Model file for the job. Use its own axes, mm. Face numbers are marked on the shaded views. A direction names the side the tool comes from. Round coordinates to 2 decimals unless told otherwise and drop trailing zeros. Loops run counter-clockwise (first coordinate to the right, second up) from the corner with the lowest first, then second, coordinate; pieces in that order, holes last. Notation, with made-up numbers: M 20,-2 L 44,-2 A27 cw 44,34 Z; hole C -18,85.5 d4. An arc over 180 degrees is marked long. Use a Markdown table: item, result. Add a question column.
Q1. Tool access for the marked faces 1 and 2: list every direction of +Z, -Z, +X, -X, +Y, -Y with a clear straight run to the whole face (end or side of a thin tool).
Q2. Mould opens along Y. For the marked faces 3, 4 and 5 say: +Y half, -Y half, draft (parallel to the pull), parting line (faces both ways), or undercut.
Q3. Probe line 1 (X direction, y = 1.3, z = 0); line 2 (Y direction, x = 1.5, z = -0.25); line 3 (Y direction, x = -1.7, z = 2.5). List the from-to ranges inside material, lowest first. Write a range as from..to.
Q4. Cut at B-B (z = 0). Give the cut face in (x, y) (3 decimals), plus the area to 3 significant figures.
Q5. Cut at C-C (y = 0.5). Give the cut face in (x, z).
Q6. Cut at D-D (z = -3). Give the cut face in (x, y).
Q7. Pin check, flat tips, straight feed: pin 1 (0.9 mm diameter, centred on x = 2, z = -3, fed in from +Y); pin 2 (2 mm diameter, centred on x = 1, y = 0.5, fed in from +Z). Stop position of each tip, or through.
Autodesk Inventor part; units mm, degrees
ref_plane "to_actuator_XY" through (0, 0, 0) normal (0, -1, 0) x (1, 0, 0)
ref_plane "to_actuator_YZ" through (0, 0, 0) normal (1, 0, 0) x (0, 0, 1)
ref_plane "to_actuator_ZX" through (0, 0, 0) normal (0, 0, 1) x (0, -1, 0)
sketch "Sketch_1" plane through (0, 0, 0) normal (0, 1, 0) x (-1, 0, 0)
  line L0 (2.2479, 3.5052) -> (-2.2479, 3.5052)
  line L1 (-2.2479, 3.5052) -> (-2.2479, -3.5052)
  line L2 (-2.2479, -3.5052) -> (2.2479, -3.5052)
  line L3 (2.2479, -3.5052) -> (2.2479, 3.5052)
extrude "Extrusion1" add sketch "Sketch_1" against normal blind 5.4102
sketch "Sketch_2" plane through (0, 0, 0) normal (0, 0, 1) x (1, 0, 0)
  line L0 (-2.2479, -0.7874) -> (-1.9456, 0)
  line L1 (-1.9456, 0) -> (1.9456, 0)
  line L2 (1.9456, 0) -> (2.2479, -0.7874)
  line L3 (2.2479, -0.7874) -> (2.2479, 0.127)
  line L4 (2.2479, 0.127) -> (-2.2479, 0.127)
  line L5 (-2.2479, 0.127) -> (-2.2479, -0.7874)
extrude "Extrusion2" cut sketch "Sketch_2" along normal mid plane 7.0104
sketch "Sketch_3" plane through (0, 0, 0) normal (1, 0, 0) x (0, 1, 0)
  line L0 (-0.7874, 3.5052) -> (0, 3.2029)
  line L1 (0, 3.2029) -> (0, -3.2029)
  line L2 (0, -3.2029) -> (-0.7874, -3.5052)
  line L3 (-0.7874, -3.5052) -> (0.127, -3.5052)
  line L4 (0.127, -3.5052) -> (0.127, 3.5052)
  line L5 (0.127, 3.5052) -> (-0.7874, 3.5052)
extrude "Extrusion3" cut sketch "Sketch_3" along normal mid plane 4.4958
sketch "Sketch_4" plane through (0, -0.9906, 0) normal (0, 1, 0) x (1, 0, 0)
  line L0 (-2.5256, 3.7556) -> (-2.5256, -3.7297)
  line L1 (-2.5256, -3.7297) -> (2.532, -3.7297)
  line L2 (2.532, -3.7297) -> (2.532, 3.7556)
  line L3 (2.532, 3.7556) -> (-2.5256, 3.7556)
  line L4 (-2.2479, 2.3368) -> (-2.2479, -2.3368)
  line L5 (-2.2479, -2.3368) -> (-1.0668, -2.3368)
  line L6 (-1.0668, -2.3368) -> (-1.0668, -3.5052)
  line L7 (-1.0668, -3.5052) -> (1.0668, -3.5052)
  line L8 (1.0668, -3.5052) -> (1.0668, -2.3368)
  line L9 (1.0668, -2.3368) -> (2.2479, -2.3368)
  line L10 (2.2479, -2.3368) -> (2.2479, 2.3368)
  line L11 (2.2479, 2.3368) -> (1.0668, 2.3368)
  line L12 (1.0668, 2.3368) -> (1.0668, 3.5052)
  line L13 (1.0668, 3.5052) -> (-1.0668, 3.5052)
  line L14 (-1.0668, 3.5052) -> (-1.0668, 2.3368)
  line L15 (-1.0668, 2.3368) -> (-2.2479, 2.3368)
extrude "Extrusion4" cut sketch "Sketch_4" along normal mid plane 0.4318
sketch "Sketch_5" plane through (0, 0, 0) normal (1, 0, 0) x (0, 1, 0)
  line L0 (0, 0) -> (1.6002, 0)
  line L1 (0.635, 0) -> (0.635, -1.1176)
  line L2 (0.635, -1.1176) -> (1.6002, -1.1176)
  line L3 (1.6002, -1.1176) -> (1.6002, -1.7399)
  line L4 (1.6002, -1.7399) -> (1.3462, -1.9939)
  line L5 (1.3462, -1.9939) -> (0, -1.9939)
  line L6 (0, -1.9939) -> (0, 0)
  line L7 (0, 0) -> (0.635, 0)
revolve "Revolution1" add sketch "Sketch_5" angle 360 about axis through (0, 0, 0) along (0, -1, 0)
sketch "Sketch_6" plane through (0, -5.4102, 0) normal (0, 1, 0) x (1, 0, 0)
  line L0 (-2.6354, 3.6285) -> (-2.6354, -3.6285)
  line L1 (-2.6354, -3.6285) -> (2.6743, -3.6285)
  line L2 (2.6743, -3.6285) -> (2.6743, 3.6285)
  line L3 (2.6743, 3.6285) -> (-2.6354, 3.6285)
  line L4 (-2.2479, -3.5052) -> (2.2479, -3.5052)
  line L5 (2.2479, -3.5052) -> (2.2479, -2.6162)
  line L6 (2.2479, -2.6162) -> (1.7399, -2.6162)
  line L7 (1.7399, -2.6162) -> (1.7399, -2.1082)
  line L8 (1.7399, -2.1082) -> (2.2479, -2.1082)
  line L9 (2.2479, -2.1082) -> (2.2479, 3.5052)
  line L10 (2.2479, 3.5052) -> (-2.2479, 3.5052)
  line L11 (-2.2479, 3.5052) -> (-2.2479, -2.1082)
  line L12 (-2.2479, -2.1082) -> (-1.7399, -2.1082)
  line L13 (-1.7399, -2.1082) -> (-1.7399, -2.6162)
  line L14 (-1.7399, -2.6162) -> (-2.2479, -2.6162)
  line L15 (-2.2479, -2.6162) -> (-2.2479, -3.5052)
extrude "Extrusion5" cut sketch "Sketch_6" along normal blind 0.4572
sketch "Sketch_7" plane through (0, -5.4102, 0) normal (0, 1, 0) x (1, 0, 0)
  line L0 (-1.8669, 2.8702) -> (-1.8669, -2.8702)
  arc A0 (-1.8669, -2.8702) -> (-1.6129, -3.1242) centre (-1.6129, -2.8702) ccw
  line L1 (-1.6129, -3.1242) -> (1.6129, -3.1242)
  arc A1 (1.6129, -3.1242) -> (1.8669, -2.8702) centre (1.6129, -2.8702) ccw
  line L2 (1.8669, -2.8702) -> (1.8669, 2.8702)
  arc A2 (1.8669, 2.8702) -> (1.6129, 3.1242) centre (1.6129, 2.8702) ccw
  line L3 (1.6129, 3.1242) -> (-1.6129, 3.1242)
  arc A3 (-1.6129, 3.1242) -> (-1.8669, 2.8702) centre (-1.6129, 2.8702) ccw
extrude "Extrusion6" cut sketch "Sketch_7" along normal blind 0.0508
sketch "Sketch_11" plane through (0, 1.6002, 0) normal (0, 1, 0) x (1, 0, 0)
  line L0 (-0.1905, -1.7145) -> (-0.1905, -2.0955)
  line L1 (-0.1905, -2.0955) -> (0.1905, -2.0955)
  line L2 (0.1905, -2.0955) -> (0.1905, -1.7145)
  line L3 (0.1905, -1.7145) -> (-0.1905, -1.7145)
extrude "Extrusion7" cut sketch "Sketch_11" against normal blind 0.254
sketch "Sketch_13" plane through (0, 0, 0) normal (0, 0, 1) x (1, 0, 0)
  line L0 (-1.143, -3.81) -> (-1.143, -4.572)
  line L1 (-1.143, -4.572) -> (1.143, -4.572)
  line L2 (1.143, -4.572) -> (1.143, -3.81)
  line L3 (1.143, -3.81) -> (-1.143, -3.81)
extrude "Extrusion8" cut sketch "Sketch_13" along normal mid plane 15.24
sketch "Sketch_14" plane through (0, 0, 0) normal (1, 0, 0) x (0, 1, 0)
  line L0 (-4.3688, 3.4544) -> (-4.572, 3.4544)
  line L1 (-4.572, 3.4544) -> (-4.572, -3.4544)
  line L2 (-4.572, -3.4544) -> (-4.3688, -3.4544)
  line L3 (-4.3688, -3.4544) -> (-3.81, -3.1318)
  line L4 (-3.81, -3.1318) -> (-3.81, 3.1318)
  line L5 (-3.81, 3.1318) -> (-4.3688, 3.4544)
extrude "Extrusion9" add sketch "Sketch_14" along normal mid plane 2.286
ref_plane "to_actuator_XY" through (0, 0, 0) normal (0, -1, 0) x (1, 0, 0)
ref_plane "to_actuator_YZ" through (0, 0, 0) normal (1, 0, 0) x (0, 0, 1)
ref_plane "to_actuator_ZX" through (0, 0, 0) normal (0, 0, 1) x (0, -1, 0)
ref_plane "to_dummy_XY" through (0, 0, 0) normal (0, -1, 0) x (1, 0, 0)
ref_plane "to_dummy_YZ" through (0, 0, 0) normal (1, 0, 0) x (0, 0, 1)
ref_plane "to_dummy_ZX" through (0, 0, 0) normal (0, 0, 1) x (0, -1, 0)
ref_plane "to_trmnl_hold_XY" through (0, -0.9906, 0) normal (0, 1, 0) x (1, 0, 0)
ref_plane "to_trmnl_hold_YZ" through (0, -0.9906, 0) normal (1, 0, 0) x (0, 0, -1)
ref_plane "to_trmnl_hold_ZX" through (0, -0.9906, 0) normal (0, 0, -1) x (0, 1, 0)
ref_plane "to_trmnls_XY" through (0, -4.9022, 0) normal (0, 1, 0) x (1, 0, 0)
ref_plane "to_trmnls_YZ" through (0, -4.9022, 0) normal (1, 0, 0) x (0, 0, -1)
ref_plane "to_trmnls_ZX" through (0, -4.9022, 0) normal (0, 0, -1) x (0, 1, 0)
properties part number "GP-body"
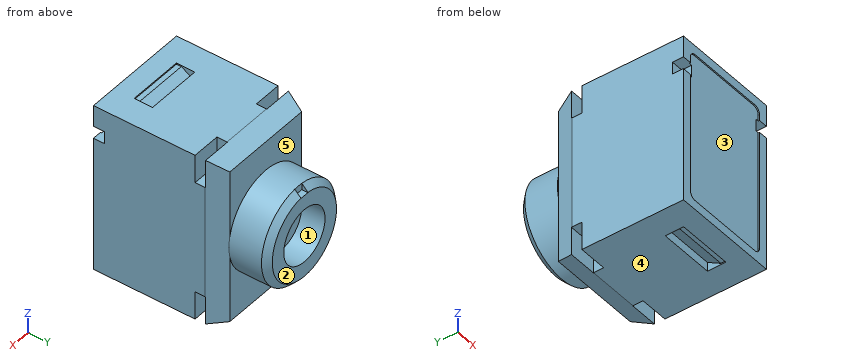
Checked values:
| question | item | result |
|---|---|---|
| 1 | face 1 | +Y |
| 1 | face 2 | +Z, -Z, +X, -X, +Y |
| 2 | face 3 | -Y half |
| 2 | face 4 | draft |
| 2 | face 5 | +Y half |
| 3 | line 1 | x = -1.99..-1.12, 1.12..1.99 |
| 3 | line 2 | y = -5.36..1.6 |
| 3 | line 3 | y = -5.36..-1.21, -0.77..0 |
| 4 | outline | M -2.248,-5.41 L -1.867,-5.41 L -1.867,-5.359 L 1.867,-5.359 L 1.867,-5.41 L 2.248,-5.41 L 2.248,-0.787 L 1.946,0 L 1.994,0 L 1.994,1.346 L 1.74,1.6 L 1.118,1.6 L 1.118,0.635 L -1.118,0.635 L -1.118,1.6 L -1.74,1.6 L -1.994,1.346 L -1.994,0 L -1.946,0 L -2.248,-0.787 Z |
| 4 | area | 28.1 mm^2 |
| 5 | outline | C 0,0 d3.99 |
| 6 | outline | M -2.25,-5.41 L -1.83,-5.41 L -1.83,-5.36 L 1.83,-5.36 L 1.83,-5.41 L 2.25,-5.41 L 2.25,-1.21 L 1.07,-1.21 L 1.07,-0.77 L 2.24,-0.77 L 1.95,0 L -1.95,0 L -2.24,-0.77 L -1.07,-0.77 L -1.07,-1.21 L -2.25,-1.21 Z |
| 7 | pin 1 | stops at y = 0 |
| 7 | pin 2 | stops at z = 3.39 |
